Source: CAD feature listing. Evaluate the final solid. Frame: model axes, mm. A direction names the side the tool comes from. Give positions to 0.01 mm unless a question says otherwise; leave off trailing zeros. Order: outer loops, then holes, each group sorted by start corner. A loop starts at its lowest first (then second) coordinate and runs counter-clockwise, first axis right, second up. Notation, with made-up numbers: (85, -40) -> (134, -40) arc R14 cw to (134, -17) -> close; hole circle Ø3 at (64.25, -1.5). An arc over 180 degrees is marked (long way). Use CSV: the item, a comma, the result in double quotes.
```python
from build123d import *

# Parameters (mm, degrees)
F3_R     = 21.863544
F4_DEPTH = 6
F5_SIZE  = 5


with BuildPart() as f2:
    # F1 (on Right) → F2 (revolve)
    with BuildSketch(Plane.YZ):
        with BuildLine():
            Line((0, 4), (0, -25))
            Line((0, -25), (6, -25))
            Line((6, -25), (7, -24))
            Line((7, -24), (7, 0))
            Line((7, 0), (20, 0))
            Line((20, 0), (20, 1.5))
            ThreePointArc((20, 1.5), (19.853553, 1.853553), (19.5, 2))
            Line((19.5, 2), (19.5, 5.322876))
            ThreePointArc((19.5, 5.322876), (18.822876, 5.822876), (18, 6))
            Line((18, 6), (16.5, 6))
            Line((16.5, 6), (9.837409, 4))
            Line((9.837409, 4), (0, 4))
        make_face()
    revolve(axis=Axis((0, 0, -10.5), (0, 0, -1)))

    # F3 (on offset) → F4 (cut)
    with BuildSketch(Plane.XY.offset(2)):
        Circle(F3_R)
        Polygon((-19.918584, 0), (-9.959292, 17.25), (9.959292, 17.25), (19.918584, 0), (9.959292, -17.25), (-9.959292, -17.25), align=None, mode=Mode.SUBTRACT)
    extrude(amount=F4_DEPTH, mode=Mode.SUBTRACT)

    # F5
    f5_edges = [f2.edges().sort_by_distance(p)[0] for p in [
        (0, -7, 0),
    ]]
    chamfer(f5_edges, length=F5_SIZE)


solid = f2.part
```
1. Section query C-C on z = -1.5. Return loops of the section in (x, y), plus the area to 3 significant figures.
Answer below:
outline,"circle Ø21 at (0, 0)"
area,"346 mm²"
2. Pin query (flat end, axial travel): P1, Ø4, axis at y = 8, z = -13.5, coming from the +X side; P2, Ø12, axis at x = 10, y = -1.5, coming from the -Z side; P3, Ø1, axis at x = 6.5, z = -17.5, coming from the -Y side; P4, Ø4.5, axis at x = -16.5, y = 10.5, coming from the +Z side. Return the tip coordinate at first contact, or that it passes through.
Answer below:
P1,"stops at x = 3.61"
P2,"stops at z = -25"
P3,"stops at y = -3.61"
P4,"stops at z = 2"
3. Access query for faces 1 (the flat face through (-15.003, 8.515, 3.972)), 2 (the flat face through (-14.875, -8.735, 3.972)). Directions: +Z, -Z, +X, -X, +Y, -Y. A direction counts if a zero-diameter tool reaches every point of the face in a straight line with its end or side. Return the directions, or none.
Answer below:
face 1,"+Z, -X, +Y"
face 2,"+Z, -X, -Y"
4. Section query A-A on y = 0. Return loops of the section in (x, z), plus the area to 3 significant figures.
Answer below:
outline,"(-20, 0) -> (-12, 0) -> (-7, -5) -> (-7, -24) -> (-6, -25) -> (6, -25) -> (7, -24) -> (7, -5) -> (12, 0) -> (20, 0) -> (20, 1.5) arc R0.5 ccw to (19.5, 2) -> (19.5, 5.32) arc R2 ccw to (18, 6) -> (16.5, 6) -> (9.84, 4) -> (-9.84, 4) -> (-16.5, 6) -> (-18, 6) arc R2 ccw to (-19.5, 5.32) -> (-19.5, 2) arc R0.5 ccw to (-20, 1.5) -> close"
area,"557 mm²"
5. Ray query, line 1 along X through (y, z) = (0, 1.5); line 2 along Z through (x, y) = (-11, 14.5); line 3 along Y through (x, z) = (-2, 3.5). Return the intervals inside material, ascending.
Answer below:
line 1,"x = -20 to 20"
line 2,"z = 0 to 5.99"
line 3,"y = -17.25 to 17.25"
6. Section query D-D on z = -11.5. Return loops of the section in (x, y).
Answer below:
outline,"circle Ø14 at (0, 0)"
7. Section query B-B on x = 0. Return loops of the section in (y, z), plus the area to 3 significant figures.
Answer below:
outline,"(-20, 0) -> (-12, 0) -> (-7, -5) -> (-7, -24) -> (-6, -25) -> (6, -25) -> (7, -24) -> (7, -5) -> (12, 0) -> (20, 0) -> (20, 1.5) arc R0.5 ccw to (19.5, 2) -> (17.25, 2) -> (17.25, 6) -> (16.5, 6) -> (9.84, 4) -> (-9.84, 4) -> (-16.5, 6) -> (-17.25, 6) -> (-17.25, 2) -> (-19.5, 2) arc R0.5 ccw to (-20, 1.5) -> close"
area,"539 mm²"
